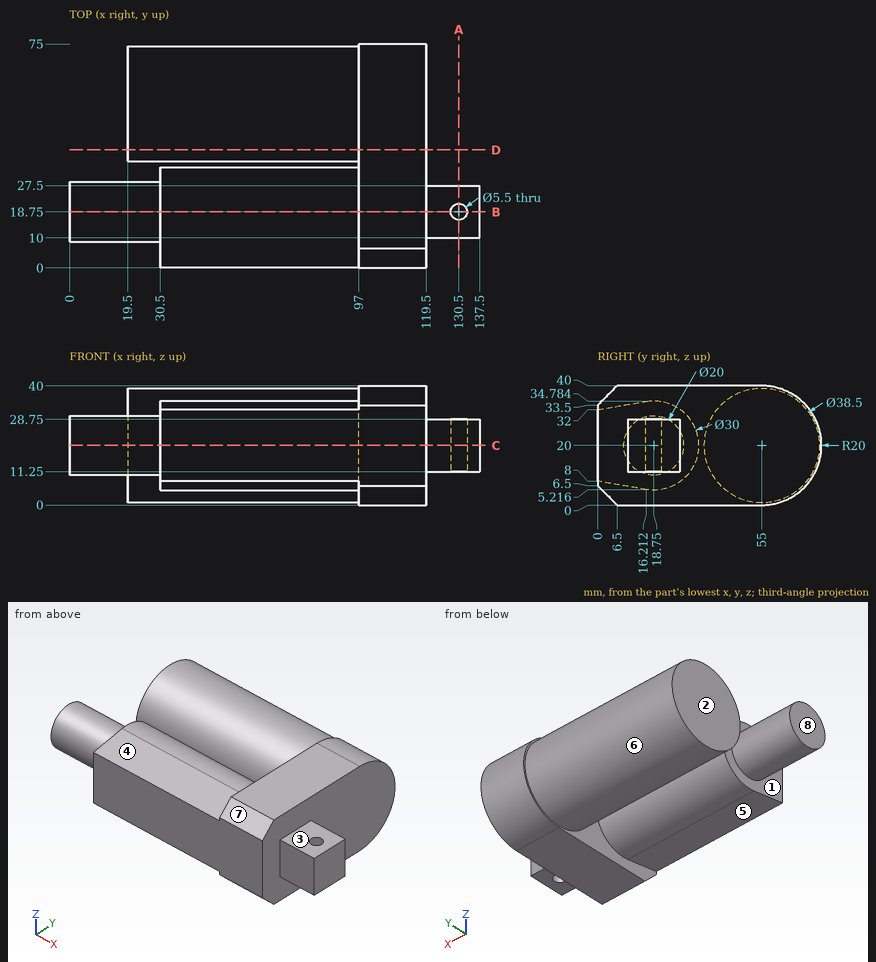
Geometry check sheet. Reference: drawing and pictorial views, mm from the part's lowest x, y, z. A direction names the side the tool comes from. Give positions to 0.01 mm unless a question says otherwise; leave off trailing zeros. Order: outer loops, then holes, each group sorted by start corner. A loop starts at its lowest first (then second) coordinate and runs counter-clockwise, first axis right, second up. Notation, with made-up numbers: (77, 85.25) -> (100, 85.25) arc R14 cw to (100, 106.25) -> close; hole circle Ø8 at (35, 56). An arc over 180 degrees is marked (long way). Use CSV: the item, a comma, the result in double quotes. Start each with the question number.
1) Go/stop test with flat-tipped pins: P1, Ø5, axis at x = 125.5, y = 16, coming from the +Z side; P2, Ø9, axis at y = 23, z = 19, coming from the -X side; P3, Ø3, axis at x = 41.5, z = 5.5, coming from the +Y side; P4, Ø6, axis at x = 44, y = 14, coming from the -Z side. Record where each tip stops, or that it passes through.
2) Set-up check for the marked faces 1, 2, 3, 4 and 5: record each of +Z, -Z, +X, -X, +Y, -Y from which the full face is reachable in a straight line by a thin tool's end or side.
3) Mould release check, pull along Y, two halves, no side actions. Record for the marked faces 6, 7 and 8: released by +Y, released by -Y, zero draft, split by the parting line, or undercut.
4) Sectioned sample at D-D, the plane y = 39.5. Record the boundary of the cut face in (x, z) (1 decimal), plus the area to 3 significant figures.
5) Sectioned sample at B-B, the plane y = 18.75. Record the boundary of the cut face in (x, z), plus the area to 3 significant figures.
6) Sectioned sample at A-A, the plane x = 130.5. Record the boundary of the cut face in (y, z).
7) Material ranges on line 1 (Y direction, x = 130.5, z = 21.5); line 2 (X direction, y = 18.75, z = 25.25); line 3 (X direction, y = 43, z = 8.5), recorded low to high. Write a range as from..to.
8) Sectioned sample at C-C, the plane z = 20. Record the boundary of the cut face in (x, y).
Recorded:
1,P1,"z = 28.75"
1,P2,"x = 0"
1,P3,"y = 69.2"
1,P4,"z = 5.1"
2,face 1,"-X"
2,face 2,"+Z, -Z, -X, +Y"
2,face 3,"+Z, +X, +Y, -Y"
2,face 4,"+Z, -X, -Y"
2,face 5,"-Z, -X, -Y"
3,face 6,"undercut"
3,face 7,"released by -Y"
3,face 8,"zero draft"
4,outline,"(19.5, 8.6) -> (97, 8.6) -> (97, 0) -> (119.5, 0) -> (119.5, 40) -> (97, 40) -> (97, 31.4) -> (19.5, 31.4) -> close"
4,area,"2,670 mm2"
5,outline,"(0, 10) -> (30.5, 10) -> (30.5, 5) -> (97, 5) -> (97, 0) -> (119.5, 0) -> (119.5, 11.25) -> (127.75, 11.25) -> (127.75, 28.75) -> (119.5, 28.75) -> (119.5, 40) -> (97, 40) -> (97, 35) -> (30.5, 35) -> (30.5, 30) -> (0, 30) -> close; (133.25, 11.25) -> (137.5, 11.25) -> (137.5, 28.75) -> (133.25, 28.75) -> close"
5,area,"3,720 mm2"
6,outline,"(10, 11.25) -> (16, 11.25) -> (16, 28.75) -> (10, 28.75) -> close; (21.5, 11.25) -> (27.5, 11.25) -> (27.5, 28.75) -> (21.5, 28.75) -> close"
7,line 1,"10..16, 21.5..27.5"
7,line 2,"0..127.75, 133.25..137.5"
7,line 3,"19.5..119.5"
8,outline,"(0, 8.75) -> (30.5, 8.75) -> (30.5, 0) -> (119.5, 0) -> (119.5, 10) -> (137.5, 10) -> (137.5, 27.5) -> (119.5, 27.5) -> (119.5, 75) -> (97, 75) -> (97, 74.25) -> (19.5, 74.25) -> (19.5, 35.75) -> (97, 35.75) -> (97, 33.75) -> (30.5, 33.75) -> (30.5, 28.75) -> (0, 28.75) -> close; hole circle Ø5.5 at (130.5, 18.75)"
